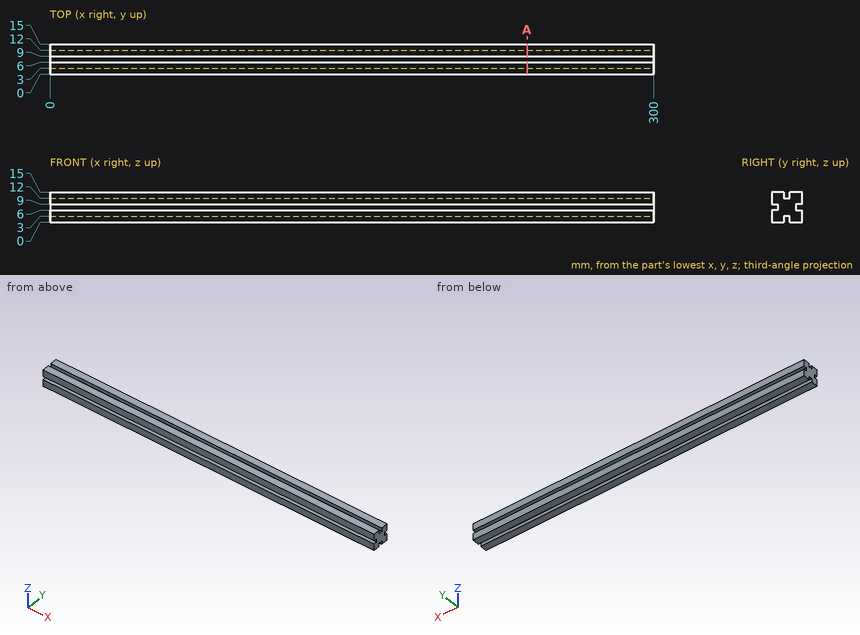
Geometry: see drawing. Coordinates: mm, zero at the bounding-box minimum. Give positions to 0.01 mm unless a question says otherwise; leave off trailing zeros. Order: outer loops, then holes, each group sorted by start corner. A loop starts at its lowest first (then second) coordinate and runs counter-clockwise, first axis right, second up. Notation, with made-up numbers: (18.25, 27.25) - (60.25, 27.25) arc R10 ccw to (60.25, 42.25) - close; hole circle Ø3 at (-37, -26). An arc over 180 degrees is marked (long way). One line per item, written item: value.
1. Line query: probe 1 along Z at (x, y) = (49, 2); probe 2 along Z at (x, y) = (256.5, 7). Output: solid intervals per line, ascending.
Determined:
probe 1: 0 to 6, 9 to 15
probe 2: 3 to 12
2. Cut plane A-A, the plane x = 237. Output: boundary loops of the cut face in (y, z).
Determined:
outline: (0, 0) - (6, 0) - (6, 3) - (9, 3) - (9, 0) - (15, 0) - (15, 6) - (12, 6) - (12, 9) - (15, 9) - (15, 15) - (9, 15) - (9, 12) - (6, 12) - (6, 15) - (0, 15) - (0, 9) - (3, 9) - (3, 6) - (0, 6) - close
3. Pin query (flat end, axial travel): pin 1 Ø1.5 at (x, y) = (169.5, 7) entering from -Z. Return the tip coordinate at first contact, or that it passes through.
Determined:
pin 1: z = 3
